```python
from build123d import *

# Parameters (mm, degrees)
F1_DEPTH  = 285.75
F2_W      = 229.616
F2_H      = 5.08
F3_DEPTH  = 6.35
F4_W      = 229.616
F4_H      = 5.334
F5_DEPTH  = 6.35
F6_R      = 1.4224
F7_DEPTH  = 11.1125
F8_W      = 12.192
F8_H      = 12.7254
F9_DEPTH  = 25.4
F12_DEPTH = 9.525
F13_R     = 1.778
F14_DEPTH = 1.6002
F15_R     = 1.905
F16_DEPTH = 1.6002
F17_R     = 2.7813
F18_DEPTH = 1.6002


with BuildPart() as f1:
    # F0 (on Top) → F1 (new body)
    with BuildSketch(Plane.XY):
        Polygon((0, 1.6002), (0, 0), (50.292, 0), (50.292, 1.6002), (1.602396, 1.6002), (1.872637, 6.756705), (4.7498, 11.379061), (4.7498, 231.2162), (3.1496, 231.2162), (3.1496, 11.8364), (0.296211, 7.252239), align=None)
    extrude(amount=F1_DEPTH)

    # F2 (on Right) → F3 (cut)
    with BuildSketch(Plane.YZ):
        with Locations((116.4082, 2.54)):
            Rectangle(F2_W, F2_H)
    extrude(amount=F3_DEPTH, mode=Mode.SUBTRACT)

    # F4 (on Right) → F5 (cut)
    with BuildSketch(Plane.YZ):
        with Locations((116.4082, 283.083)):
            Rectangle(F4_W, F4_H)
    extrude(amount=F5_DEPTH, mode=Mode.SUBTRACT)

    # F6 (on face) → F7 (join)
    with BuildSketch(Plane.YZ.offset(4.7498)):
        with Locations((154.0002, 248.285)):
            Circle(F6_R)
        with Locations((19.1262, 249.555)):
            Circle(F6_R)
        with Locations((121.285, 100.965)):
            Circle(F6_R)
        with Locations((20.4216, 90.1446)):
            Circle(F6_R)
        with Locations((41.275, 100.965)):
            Circle(F6_R)
        with Locations((20.4216, 19.1516)):
            Circle(F6_R)
    extrude(amount=F7_DEPTH)

    # F8 (on face) → F9 (cut)
    with BuildSketch(Plane.YZ.offset(4.7498)):
        with Locations((182.0291, 89.3699)):
            Rectangle(F8_W, F8_H)
    extrude(amount=-F9_DEPTH, mode=Mode.SUBTRACT)

    # F11 (on offset) → F12 (join)
    with BuildSketch(Plane.XY.offset(84.7344)):
        with BuildLine():
            Line((14.2748, 176.7332), (14.2748, 178.3334))
            Line((14.2748, 178.3334), (4.7498, 178.3334))
            ThreePointArc((4.7498, 178.3334), (3.618288, 177.864712), (3.1496, 176.7332))
            Line((3.1496, 176.7332), (3.1496, 175.9331))
            Line((3.1496, 175.9331), (4.7498, 175.9331))
            ThreePointArc((4.7498, 175.9331), (4.984144, 176.498856), (5.5499, 176.7332))
            Line((5.5499, 176.7332), (14.2748, 176.7332))
        make_face()
    extrude(amount=F12_DEPTH)

    # F13 (on face) → F14 (cut, through all)
    with BuildSketch(Plane(origin=(0, 178.3334, 0), x_dir=(-1, 0, 0), z_dir=(0, 1, 0))):
        with Locations((-8.9916, 89.5096)):
            Circle(F13_R)
    extrude(amount=-F14_DEPTH, mode=Mode.SUBTRACT)

    # F15 (on face) → F16 (cut, through all)
    with BuildSketch(Plane.XZ):
        with Locations((12.065, 134.112)):
            Circle(F15_R)
        with Locations((17.145, 134.112)):
            Circle(F15_R)
        with Locations((12.065, 129.667)):
            Circle(F15_R)
        with Locations((17.145, 129.667)):
            Circle(F15_R)
    extrude(amount=-F16_DEPTH, mode=Mode.SUBTRACT)

    # F17 (on face) → F18 (cut, through all)
    with BuildSketch(Plane.XZ):
        with Locations((25.4254, 7.112)):
            Circle(F17_R)
        with Locations((25.4254, 278.638)):
            Circle(F17_R)
    extrude(amount=-F18_DEPTH, mode=Mode.SUBTRACT)


solid = f1.part
```
Geometry check sheet. Reference: the model listing, model coordinates, mm. Give positions to 0.01 mm unless a question says otherwise; leave off trailing zeros. Loops run counter-clockwise (first coordinate to the right, second up) from the corner with the lowest first, then second, coordinate; pieces in that order, holes last. Notation, with made-up numbers: M 1,17.5 L 26,17.5 A28 ccw 26,56.5 Z; hole C -11,-2.75 d7. An arc over 180 degrees is marked long. Write item = value, one per line. Start each with the question number.
1. Go/stop test with flat-tipped pins: P1, Ø3, axis at y = 41.5, z = 100.5, coming from the +X side; P2, Ø1.5, axis at y = 184.5, z = 196, coming from the -X side; P3, Ø2.5, axis at x = 12.065, z = 134.112, coming from the +Y side (3 decimals); P4, Ø9, axis at x = 25.43, z = 278.64, coming from the +Y side. Record where each tip stops, or that it passes through.
2. Draft check along Y on faces 1 (the face through (11, 176.733, 89)), 2 (the face through (25, 0, 141)), 3 (the face through (11, 178.333, 90)). Enter one of: +Y half, -Y half, draft (parallel to the pull), parting line (faces both ways), or undercut.
3. Thickness scan on probe 1 along X at (y, z) = (212, 184.5); probe 2 along Y at (x, z) = (45, 132); probe 3 along Z at (x, y) = (11, 41). Record the ranges inside material, lowest first.
4. Section check B-B, the plane y = 135.5. Enter the section's corners in (x, z).
5. Section check A-A, the plane z = 34. Enter the section's corners in (x, y), plus the area to 3 significant figures.
Values follow:
q1.P1 = 15.86
q1.P2 = 3.15
q1.P3 = through
q1.P4 = 1.6
q2.face_1 = undercut
q2.face_2 = -Y half
q2.face_3 = +Y half
q3.probe_1 = 3.15 to 4.75
q3.probe_2 = 0 to 1.6
q3.probe_3 = 99.57 to 102.36
q4.outline = M 3.15,5.08 L 4.75,5.08 L 4.75,280.42 L 3.15,280.42 Z
q5.outline = M 0,0 L 50.29,0 L 50.29,1.6 L 1.6,1.6 L 1.87,6.76 L 4.75,11.38 L 4.75,231.22 L 3.15,231.22 L 3.15,11.84 L 0.3,7.25 L 0,1.6 Z
q5.area = 449 mm^2
